Solid Edge part; units mm, degrees
sketch "Sketch1" plane through (0, 0, 0) normal (0, 0, 1) x (1, 0, 0)
  circle A0 centre (0, 0) radius 11
extrude "Protrusion1" add sketch "Sketch1" along normal mid plane 200
sketch "Sketch2" plane through (0, 0, 100) normal (0, 0, 1) x (1, 0, 0)
  circle A0 centre (0, 0) radius 9
extrude "Cutout1" cut sketch "Sketch2" against normal up to vertex (200 mm away)
sketch "Sketch3" plane through (0, 0, 0) normal (0, -1, 0) x (1, 0, 0)
  circle A0 centre (0, 89) radius 2.5
extrude "ExtrudedCutout_2" cut sketch "Sketch3" along normal mid plane 30
Geometry: final body of the model. Coordinates: model frame, mm. Give positions to 0.01 mm unless a question says otherwise; leave off trailing zeros. Order: outer loops, then holes, each group sorted by start corner. A loop starts at its lowest first (then second) coordinate and runs counter-clockwise, first axis right, second up. Notation, with made-up numbers: (-13, 58) -> (27, 58) arc R20 ccw to (27, 73) -> close; hole circle Ø3 at (72.25, 41). An arc over 180 degrees is marked (long way). Write each question's results on one line, items separated by ' | '. Start each with the question number.
1) Draft query along Z for faces 1 (the flat face through (2, -9, 100)), 2 (the flat face through (2, -9, -100)), 3 (the cylindrical face through (2.31, 9.81, 88.04)). Return one class per face: pulls with the +Z half, pulls with the -Z half, needs draft (parallel to the pull), parting line crosses it, or undercut.
2) Section C-C (x = 0). Return loops of the section in (y, z), then the cut area to 3 significant figures.
3) Section B-B (z = 89). Return loops of the section in (x, y).
4) Section D-D (z = -40). Return loops of the section in (x, y).
5) Line query: line 1 (Z direction, x = 0, y = -9.7); line 2 (Y direction, x = -0.75, z = -3); line 3 (Y direction, x = -7, z = 87). Output: solid intervals per line, ascending. Write a range as from..to.
6) First-contact query: pin 1 (4 mm diameter, centred on x = 0, z = 89, fed in from -Y); pin 2 (12 mm diameter, centred on x = 7, z = 69, fed in from +Y); pin 3 (1 mm diameter, centred on x = 3, z = -39.5, fed in from +Y); pin 4 (4 mm diameter, centred on y = 5.5, z = 33, fed in from +X). Flat tips, straight axial feed; report the tip coordinate or a pass-through.
7) Section A-A (y = 0). Return loops of the section in (x, z), then the cut area to 3 significant figures.
Calculated:
1) face 1: pulls with the +Z half | face 2: pulls with the -Z half | face 3: undercut
2) outline: (-11, -100) -> (-9, -100) -> (-9, 86.5) -> (-11, 86.5) -> close; (-11, 91.5) -> (-9, 91.5) -> (-9, 100) -> (-11, 100) -> close; (9, -100) -> (11, -100) -> (11, 86.5) -> (9, 86.5) -> close; (9, 91.5) -> (11, 91.5) -> (11, 100) -> (9, 100) -> close | area: 780 mm2
3) outline: (-2.5, -10.71) -> (-2.5, -8.65) arc R9 cw to (-2.5, 8.65) -> (-2.5, 10.71) arc R11 ccw to start; (2.5, -10.71) arc R11 ccw to (2.5, 10.71) -> (2.5, 8.65) arc R9 cw to (2.5, -8.65) -> close
4) outline: circle Ø22 at (0, 0); hole circle Ø18 at (0, 0)
5) line 1: -100..86.5, 91.5..100 | line 2: -10.97..-8.97, 8.97..10.97 | line 3: -8.49..-5.66, 5.66..8.49
6) pin 1: through | pin 2: y = 10.95 | pin 3: y = 10.71 | pin 4: x = 10.43
7) outline: (-11, -100) -> (-9, -100) -> (-9, 100) -> (-11, 100) -> close; (9, -100) -> (11, -100) -> (11, 100) -> (9, 100) -> close | area: 800 mm2
